Could you check a few things on this model? Use its own coordinates, in mm. Face numbers are marked on the shaded views. A direction names the side the tool comes from. Round coordinates to 2 decimals unless told otherwise and drop trailing zeros. Loops run counter-clockwise (first coordinate to the right, second up) from the corner with the lowest first, then second, coordinate; pieces in that order, holes last. Notation, with made-up numbers: M -21.5,-26 L 19.5,-26 A13 ccw 19.5,-19 Z; hole C 29.5,17.25 d1. An arc over 180 degrees is marked long. Answer in a Markdown table with one row per item.
```python
from build123d import *

# Parameters (mm, degrees)
SKETCH_1_W          = 11.5
SKETCH_1_H          = 9
EXTRUDE_1_DEPTH     = 15.5
CUT_EXTRUDE_1_REACH = 21.904
CUT_EXTRUDE_3_DEPTH = 10
SKETCH_7_R          = 1.6
CUT_EXTRUDE_4_DEPTH = 3.2
SKETCH_9_W          = 15
SKETCH_9_H          = 2.5
EXTRUDE_2_DEPTH     = 15
EXTRUDE_3_DEPTH     = 6
CUT_EXTRUDE_5_DEPTH = 25
SKETCH_12_R         = 1.55
CUT_EXTRUDE_6_DEPTH = 50
EXTRUDE_4_DEPTH     = 2


with BuildPart() as part:
    # 草图1 → 凸台-拉伸1 (new, symmetric)
    with BuildSketch(Plane(origin=(0, 0, 0), x_dir=(1, 0, 0), z_dir=(0, 1, 0))):
        with Locations((2.905437314, 1.868632411)):
            Rectangle(SKETCH_1_W, SKETCH_1_H)
    extrude(amount=EXTRUDE_1_DEPTH, both=True)

    # 草图3 → 切除-拉伸1 (cut, up to next)
    with BuildSketch(Plane.XY.offset(2.631367589), mode=Mode.PRIVATE) as cut_extrude_1_sk1:
        Polygon((-2.844562686, 15.5), (-2.844562686, 12.5), (7.496374606, 15.5), align=None)
    cut_extrude_1_tool1 = extrude(cut_extrude_1_sk1.sketch, amount=-CUT_EXTRUDE_1_REACH, mode=Mode.PRIVATE) & part.part
    # 草图3 → 切除-拉伸1 (cut, up to next)
    with BuildSketch(Plane.XY.offset(2.631367589), mode=Mode.PRIVATE) as cut_extrude_1_sk2:
        Polygon((7.496374606, -15.5), (-2.844562686, -15.5), (-2.844562686, -12.5), align=None)
    cut_extrude_1_tool2 = extrude(cut_extrude_1_sk2.sketch, amount=-CUT_EXTRUDE_1_REACH, mode=Mode.PRIVATE) & part.part
    add(cut_extrude_1_tool1.solids().sort_by_distance((0.602416, 14.5, 2.631368))[0], mode=Mode.SUBTRACT)
    add(cut_extrude_1_tool2.solids().sort_by_distance((0.602416, -14.5, 2.631368))[0], mode=Mode.SUBTRACT)

    # 草图6 → 切除-拉伸3 (cut)
    with BuildSketch(Plane.ZY.offset(2.844562686)):
        Polygon((0.631367589, 9.665706569), (-6.368632411, 9.665706569), (-11.26294246, 9.665706569), (-11.26294246, -9.665706569), (-6.368632411, -9.665706569), (0.631367589, -9.665706569), align=None)
    extrude(amount=-CUT_EXTRUDE_3_DEPTH, mode=Mode.SUBTRACT)

    # 草图7 → 切除-拉伸4 (cut)
    with BuildSketch(Plane(origin=(0, 0, 0.631367589), x_dir=(-1, 0, 0), z_dir=(0, 0, -1))):
        with Locations(Location((-4.155437314, 0, 0), (0, 0, 90))):
            Circle(SKETCH_7_R)
    extrude(amount=-CUT_EXTRUDE_4_DEPTH, mode=Mode.SUBTRACT)

    # 草图9 → 凸台-拉伸2 (add, symmetric)
    with BuildSketch(Plane(origin=(0, 0, 0), x_dir=(1, 0, 0), z_dir=(0, 1, 0))):
        with Locations((16.155437314, 5.118632411)):
            Rectangle(SKETCH_9_W, SKETCH_9_H)
    extrude(amount=EXTRUDE_2_DEPTH, both=True)

    # 草图10 → 凸台-拉伸3 (add)
    with BuildSketch(Plane(origin=(0, 0, -6.368632411), x_dir=(-1, 0, 0), z_dir=(0, 0, -1))):
        Polygon((2.844562686, 9.665706569), (2.844562686, 15.89839332), (-8.411310933, 20.920270748), (-23.655437314, 15), (-23.655437314, -15), (-8.411310933, -20.920270748), (2.844562686, -15.89839332), (2.844562686, -9.665706569), (-7.155437314, -9.665706569), (-7.155437314, 9.665706569), align=None)
    extrude(amount=EXTRUDE_3_DEPTH)

    # 草图11 → 切除-拉伸5 (cut, symmetric)
    with BuildSketch(Plane(origin=(0, 0, 0), x_dir=(1, 0, 0), z_dir=(0, 1, 0))):
        Polygon((8.411310933, 12.368632411), (0.155437314, 10.860086612), (0.155437314, 6.368632411), (-2.844562686, 6.368632411), (-2.844562686, 10.368632411), (-2.844562686, 12.368632411), align=None)
    extrude(amount=CUT_EXTRUDE_5_DEPTH, both=True, mode=Mode.SUBTRACT)

    # 草图12 → 切除-拉伸6 (cut)
    with BuildSketch(Plane(origin=(-1.915261303, 0, -10.481720391), x_dir=(-0.9837127141080302, 0, 0.17974786814372187), z_dir=(-0.17974786814372187, 0, -0.9837127141080303))):
        with Locations((-7.219941257, 12.090668535)):
            Circle(SKETCH_12_R)
    extrude(amount=-CUT_EXTRUDE_6_DEPTH, mode=Mode.SUBTRACT)

    # 草图13 → 凸台-拉伸4 (add)
    with BuildSketch(Plane(origin=(-1.915261303, 0, -10.481720391), x_dir=(-0.9837127141080303, 0, 0.17974786814372185), z_dir=(-0.17974786814372182, 0, -0.9837127141080302))):
        Polygon((-10.497548815, 20.920270748), (-10.497548815, 16.920270748), (-2.104983078, 16.920270748), (-2.104983078, 17.23686182), align=None)
        Polygon((-10.497548815, -20.920270748), (-10.497548815, -16.920270748), (-2.104983078, -16.920270748), (-2.104983078, -17.23686182), align=None)
    extrude(amount=EXTRUDE_4_DEPTH)


solid = part.part
```
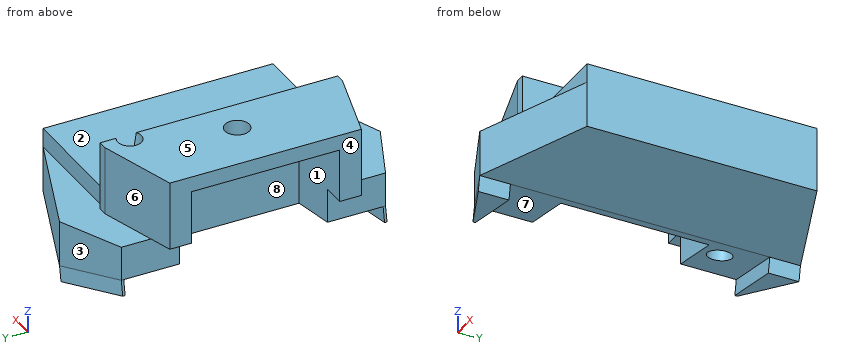
1) I want a section at D-D, the plane y = 18.5. Please give me the cut outline in (x, z), plus the area to 3 significant figures.
Computed:
| item | result |
|---|---|
| outline | M 2.63,-13.34 L 8.05,-14.34 L 8.41,-12.37 L 14.64,-12.37 L 14.64,-6.37 L 2.99,-6.37 L 2.99,-11.38 Z |
| area | 78.3 mm² |
2) I want a section at C-C, the plane y = -14. Please give me the cut outline in (x, z).
Computed:
| item | result |
|---|---|
| outline | M 0.16,-10.86 L 8.41,-12.37 L 23.66,-12.37 L 23.66,-3.87 L 8.66,-3.87 L 8.66,2.63 L 2.33,2.63 L 2.33,-6.37 L 0.16,-6.37 Z |
3) I want a section at A-A, the plane y = 0. Please give me the cut outline in (x, z).
Computed:
| item | result |
|---|---|
| outline | M -2.84,0.63 L 2.56,0.63 L 2.56,2.63 L -2.84,2.63 Z; M 5.76,0.63 L 7.16,0.63 L 7.16,-12.14 L 8.41,-12.37 L 23.66,-12.37 L 23.66,-3.87 L 8.66,-3.87 L 8.66,2.63 L 5.76,2.63 Z |
4) I need wall thicknesses on line 1 (X direction, y = 0, z = 2); line 2 (X direction, y = 8, z = -9.75); line 3 (X direction, y = -8.5, z = -1.5). Which ranges of each line are inside material? Lowest first, please.
Computed:
| item | result |
|---|---|
| line 1 | x = -2.84 to 2.56, 5.76 to 8.66 |
| line 2 | x = 7.16 to 23.66 |
| line 3 | x = 7.16 to 8.66 |
5) Which directions (+Z, -Z, +X, -X, +Y, -Y) give clear straight access to the entire face, cutting with the end or side of a thin tool? Please do the marked faces 1, 2, 3 and 4.
Computed:
| item | result |
|---|---|
| face 1 | -Z, -X |
| face 2 | +Z, +X, +Y, -Y |
| face 3 | +Z, -X, +Y |
| face 4 | +Z, -Z, -X, +Y, -Y |
6) I want a section at B-B, the plane y = -7. Please give me the cut outline in (x, z), plus the area to 3 significant figures.
Computed:
| item | result |
|---|---|
| outline | M -2.84,0.63 L 7.16,0.63 L 7.16,-12.14 L 8.41,-12.37 L 23.66,-12.37 L 23.66,-3.87 L 8.66,-3.87 L 8.66,2.63 L -2.84,2.63 Z |
| area | 170 mm² |
7) Will these pins go through, and if not, where does the flat tip stop? P1, Ø2.5, axis at x = 15, y = -16, coming from the +Z side; P2, Ø8, axis at y = 13, z = -9, coming from the -X side; P3, Ø0.6, axis at x = 8.5, z = -1.5, coming from the -Y side; P4, Ø4, axis at x = 13.5, y = 19, coming from the +Z side.
Computed:
| item | result |
|---|---|
| P1 | stops at z = -3.87 |
| P2 | stops at x = -2.84 |
| P3 | stops at y = -15.5 |
| P4 | stops at z = -6.37 |
8) If we mould it in two halves opening along Y, with no side actions, what happens to the marked faces 5, 6, 7 and 8? For each: released by +Y, released by -Y, zero draft, split by the parting line, or undercut.
Computed:
| item | result |
|---|---|
| face 5 | zero draft |
| face 6 | released by +Y |
| face 7 | undercut |
| face 8 | undercut |
